Study the drawing (mm; zero at the part's minimum x, y, z) and answer. Give positions to 0.01 mm unless a question says otherwise; leave off trailing zeros. Order: outer loops, then holes, each group sorted by start corner. A loop starts at its lowest first (then second) coordinate and runs counter-clockwise, first axis right, second up. Notation, with made-up numbers: (86, 54) -> (126, 54) arc R29 ccw to (126, 85) -> close; hole circle Ø1 at (-2.75, 55.25). An arc over 180 degrees is marked (long way). One line per question, with ' | ' between items. Start each with the question number.
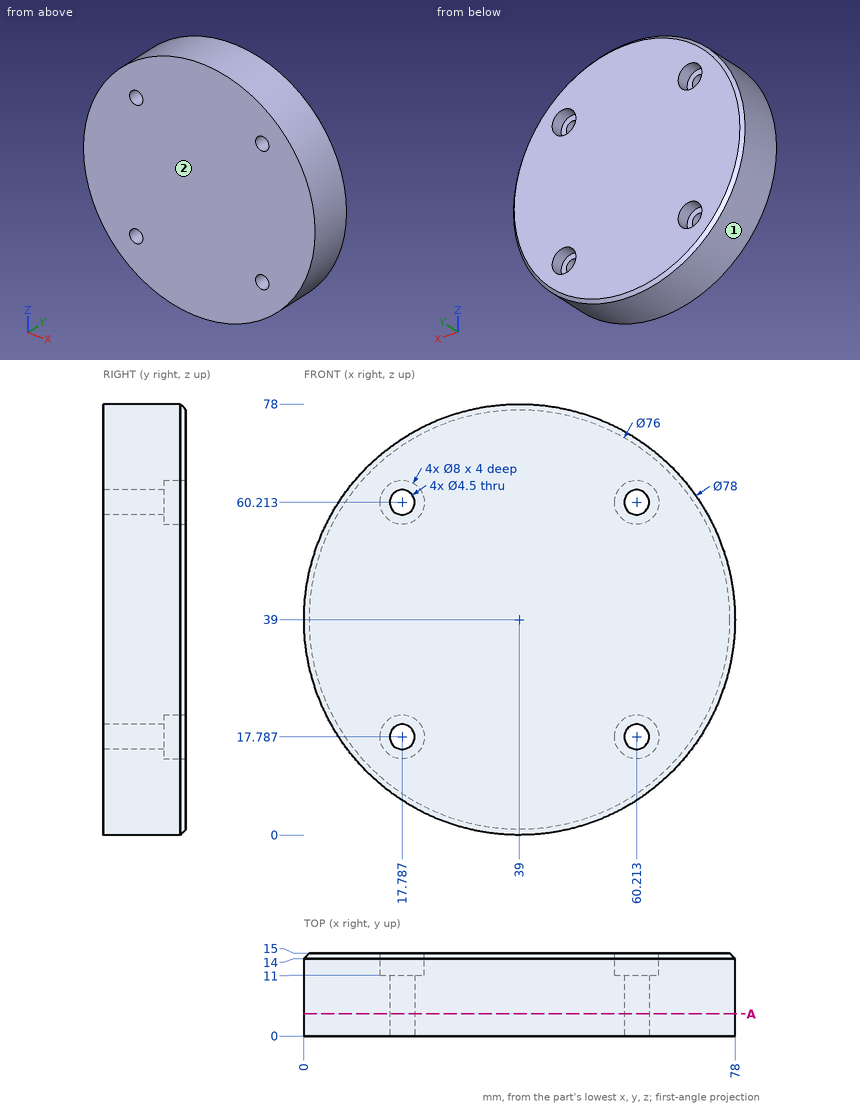
Q1. Determine the mould class of the marked faces 1 and 2 for opening direction Z: pulls with the +Z half, pulls with the -Z half, needs draft (parallel to the pull), parting line crosses it, or undercut.
Q2. Given P1, Ø3.5, axis at x = 17.79, z = 60.21, coming from the +Y side (1 decimal); P2, Ø1, axis at x = 59.5, y = 8.5, coming from the -Z side; P3, Ø2, axis at x = 10, y = 9, coming from the +Z side; P4, Ø6, axis at x = 66.5, y = 1.5, coming from the +Z side, each flat-ended and moving along its own axis, determine where each tip first touches the part or whether it passes through.
Q3. A cutting plane is placed at A-A, the plane y = 4. Determine the outline of the cut face in (x, z).
Q4. Find the intervals of material crossed by line 1 (X direction, y = 3.75, z = 17) (1 decimal); line 2 (X direction, y = 2.75, z = 62) (1 decimal); line 3 (Z direction, x = 60.5, y = 4.75) (1 decimal), in increasing order.
Geometry results:
1) face 1: parting line crosses it | face 2: needs draft
2) P1: through | P2: z = 5.52 | P3: z = 66.15 | P4: z = 69.34
3) outline: circle Ø78 at (39, 39); hole circle Ø4.5 at (17.79, 17.79); hole circle Ø4.5 at (17.79, 60.21); hole circle Ø4.5 at (60.21, 17.79); hole circle Ø4.5 at (60.21, 60.21)
4) line 1: 6.8 to 15.7, 19.9 to 58.1, 62.3 to 71.2 | line 2: 7.5 to 16.4, 19.2 to 58.8, 61.6 to 70.5 | line 3: 6.5 to 15.6, 20 to 58, 62.4 to 71.5
